Check sheet for the modelled part. Datum: model origin and axes. Units: mm. A direction names the side the tool comes from. Round coordinates to 2 decimals unless told otherwise and drop trailing zeros. Write each loop counter-clockwise with the first axis right and the second up, starting at its lowest first coordinate (ties: lowest second). Pieces come first, ordered by that corner, then holes. Notation, with made-up numbers: (13, 70.5) -> (22, 70.5) arc R36 cw to (22, 108.5) -> close; hole circle Ø3 at (-7, 86.25). An arc over 180 degrees is marked (long way). Write item = value, one per line.
Autodesk Inventor part; units mm, degrees
ref_plane "planeForCenterLineOfPowerCells" through (-12.7, 68.1014, 57.1438) normal (0, 0.766, 0.6428) x (1, 0, 0)
ref_plane "YZ Plane" through (0, 0, 0) normal (1, 0, 0) x (0, 1, 0)
ref_plane "XZ Plane" through (0, 0, 0) normal (0, 1, 0) x (-1, 0, 0)
sketch "Sketch1" plane through (0, 0, 0) normal (1, 0, 0) x (0, 1, 0)
  line L0 (0, 0) -> (0, -609.6)
  line L1 (0, -609.6) -> (511.5151, -609.6)
  line L2 (511.5151, -609.6) -> (0, 0)
  line L3 (25.4, -69.7859) -> (457.0447, -584.2)
  line L4 (457.0447, -584.2) -> (25.4, -584.2)
  line L5 (25.4, -584.2) -> (25.4, -69.7859)
  dimension "d0" = 609.6
  dimension "d1" = 40
  dimension "d2" = 25.4
  dimension "d3" = 25.4
  dimension "d4" = 25.4
extrude "Extrusion1" add sketch "Sketch1" along normal mid plane 25.4
sketch "Sketch2" plane through (12.7, 0, 0) normal (1, 0, 0) x (0, 0, -1)
  line L0 (0, 0) -> (609.6, 0)
  line L1 (0, 0) -> (610.7413, 512.4728)
  line L2 (69.7859, 25.4) -> (584.2, 457.0447)
  line L3 (68.5783, 24.3867) -> (584.2, 457.0447)
  line L4 (584.2, 457.0447) -> (609.6, 478.3578)
  line L5 (584.2, 25.4) -> (69.7859, 25.4)
  line L6 (69.7859, 25.4) -> (39.5154, 0)
  line L7 (39.5154, 0) -> (0, 0)
  line L8 (609.6, 0) -> (609.6, 511.5151)
  line L9 (609.6, 511.5151) -> (609.6, 478.3578)
  point P0 (609.6, 511.5151)
  point P1 (69.7859, 25.4)
extrude "Extrusion2" add sketch "Sketch2" along normal blind 25.4 contours L1 L8 L4 L2 L3 L6 L0
ref_plane "planeForCenterLineOfPowerCells" through (-12.7, 68.1014, 57.1438) normal (0, 0.766, 0.6428) x (1, 0, 0)
properties part number "ballRampLeftSideV04"
(1) Release check for a two-part mould opening along Y. For faces 1 (the flat face through (0, 244, -584.2)), 2 (the flat face through (1, 0, -301)), 3 (the flat face through (-12.7, 255, -326)) record: pulls with the +Y half, pulls with the -Y half, needs draft (parallel to the pull), parting line crosses it, or undercut.
Worked answers:
face_1 = undercut
face_2 = pulls with the -Y half
face_3 = needs draft
(2) Access from +Z, -Z, +X, -X, +Y, -Y to the whole of each face (thin tool, end or side, straight path). Record for faces 4 (the flat face through (12.7, 8, -450)), 5 (the flat face through (1, 252, -609.6)), 6 (the flat face through (0, 25.4, -331)).
Worked answers:
face_4 = -Z, +X, -Y
face_5 = -Z, +X, -X, +Y, -Y
face_6 = +X, -X
(3) Sectioned sample at B-B on z = -341. Enter the section's corners in (x, y).
Worked answers:
outline = (-12.7, 0) -> (12.7, 0) -> (12.7, 25.4) -> (-12.7, 25.4) -> close; (-12.7, 252.98) -> (38.1, 252.98) -> (38.1, 286.13) -> (-12.7, 286.13) -> close
(4) Sectioned sample at C-C on x = 20. Enter the section's corners in (y, z).
Worked answers:
outline = (0, -39.52) -> (24.39, -68.58) -> (457.04, -584.2) -> (478.36, -609.6) -> (511.52, -609.6) -> (0, 0) -> close
(5) Material ranges on L1, parallel to Y at x = 6.5, z = -93; L2, parallel to Z at x = 7.5, y = 207; L3, parallel to Y at x = 2, z = -316, recorded low to high. Write a range as [from, to].
Worked answers:
L1 = [0, 25.4], [44.88, 78.04]
L2 = [-609.6, -584.2], [-286.21, -246.69]
L3 = [0, 25.4], [232, 265.16]
(6) Sectioned sample at A-A on y = 190.5. Enter the section's corners in (x, z).
Worked answers:
outline = (-12.7, -609.6) -> (12.7, -609.6) -> (12.7, -584.2) -> (-12.7, -584.2) -> close; (-12.7, -266.54) -> (38.1, -266.54) -> (38.1, -227.03) -> (-12.7, -227.03) -> close
(7) Go/stop test with flat-tipped pins: P1, Ø1.5, axis at y = 370.5, z = -437.5, coming from the -X side (3 decimals); P2, Ø12.5, axis at x = 2.5, z = -275, coming from the +Y side. Record where each tip stops, or that it passes through.
Worked answers:
P1 = through
P2 = 236
